```python
from build123d import *

# Parameters (mm, degrees)
SKETCH1_R           = 1.190625
SKETCH1_R_2         = 0.79375
BOSS_EXTRUDE1_DEPTH = 1.984375
SKETCH2_R           = 3.175
CUT_EXTRUDE1_DEPTH  = 0.7493
SKETCH3_R           = 4.365625
BOSS_EXTRUDE2_DEPTH = 2.3876
SKETCH4_R           = 2.778125
CUT_EXTRUDE2_DEPTH  = 2.9591
SKETCH5_R           = 3.7703125
SKETCH5_R_2         = 3.175
BOSS_EXTRUDE3_DEPTH = 0.4572


with BuildPart() as part:
    # Sketch1 → Boss-Extrude1 (new body)
    with BuildSketch(Plane(origin=(0, 0, 0), x_dir=(1, 0, 0), z_dir=(0, 1, 0))):
        with BuildLine():
            Line((-3.96335347, 4.938233395), (-2.375942501, 13.151798758))
            ThreePointArc((-2.375942501, 13.151798758), (-0.037956575, 15.081193279), (2.300029351, 13.151798758))
            Line((2.300029351, 13.151798758), (3.933761069, 4.9618349))
            ThreePointArc((3.933761069, 4.9618349), (4.283887399, 4.309571692), (4.938233395, 3.96335347))
            Line((4.938233395, 3.96335347), (13.151798758, 2.375942501))
            ThreePointArc((13.151798758, 2.375942501), (15.081193279, 0.037956575), (13.151798758, -2.300029351))
            Line((13.151798758, -2.300029351), (4.9618349, -3.933761069))
            ThreePointArc((4.9618349, -3.933761069), (4.309571692, -4.283887399), (3.96335347, -4.938233395))
            Line((3.96335347, -4.938233395), (2.375942501, -13.151798758))
            ThreePointArc((2.375942501, -13.151798758), (0.037956575, -15.081193279), (-2.300029351, -13.151798758))
            Line((-2.300029351, -13.151798758), (-3.933761069, -4.9618349))
            ThreePointArc((-3.933761069, -4.9618349), (-4.283887399, -4.309571692), (-4.938233395, -3.96335347))
            Line((-4.938233395, -3.96335347), (-13.151798758, -2.375942501))
            ThreePointArc((-13.151798758, -2.375942501), (-15.081193279, -0.037956575), (-13.151798758, 2.300029351))
            Line((-13.151798758, 2.300029351), (-4.9618349, 3.933761069))
            ThreePointArc((-4.9618349, 3.933761069), (-4.309571692, 4.283887399), (-3.96335347, 4.938233395))
        make_face()
        Circle(SKETCH1_R, mode=Mode.SUBTRACT)
        with Locations((-0.037956575, 12.699943279)):
            Circle(SKETCH1_R_2, mode=Mode.SUBTRACT)
        with Locations((-0.031124391, 10.413953489)):
            Circle(SKETCH1_R_2, mode=Mode.SUBTRACT)
        with Locations((-0.024292208, 8.127963699)):
            Circle(SKETCH1_R_2, mode=Mode.SUBTRACT)
        with Locations((12.699943279, 0.037956575)):
            Circle(SKETCH1_R_2, mode=Mode.SUBTRACT)
        with Locations((10.413953489, 0.031124391)):
            Circle(SKETCH1_R_2, mode=Mode.SUBTRACT)
        with Locations((8.127963699, 0.024292208)):
            Circle(SKETCH1_R_2, mode=Mode.SUBTRACT)
        with Locations((0.037956575, -12.699943279)):
            Circle(SKETCH1_R_2, mode=Mode.SUBTRACT)
        with Locations((0.031124391, -10.413953489)):
            Circle(SKETCH1_R_2, mode=Mode.SUBTRACT)
        with Locations((0.024292208, -8.127963699)):
            Circle(SKETCH1_R_2, mode=Mode.SUBTRACT)
        with Locations((-12.699943279, -0.037956575)):
            Circle(SKETCH1_R_2, mode=Mode.SUBTRACT)
        with Locations((-10.413953489, -0.031124391)):
            Circle(SKETCH1_R_2, mode=Mode.SUBTRACT)
        with Locations((-8.127963699, -0.024292208)):
            Circle(SKETCH1_R_2, mode=Mode.SUBTRACT)
    extrude(amount=BOSS_EXTRUDE1_DEPTH)

    # Sketch2 → Cut-Extrude1 (cut)
    with BuildSketch(Plane(origin=(0, 1.984375, 0), x_dir=(1, 0, 0), z_dir=(0, 1, 0))):
        Circle(SKETCH2_R)
    extrude(amount=-CUT_EXTRUDE1_DEPTH, mode=Mode.SUBTRACT)

    # Sketch3 → Boss-Extrude2 (add)
    with BuildSketch(Plane.XZ):
        Circle(SKETCH3_R)
    extrude(amount=BOSS_EXTRUDE2_DEPTH)

    # Sketch4 → Cut-Extrude2 (cut)
    with BuildSketch(Plane.XZ.offset(2.3876)):
        Circle(SKETCH4_R)
    extrude(amount=-CUT_EXTRUDE2_DEPTH, mode=Mode.SUBTRACT)

    # Sketch5 → Boss-Extrude3 (add)
    with BuildSketch(Plane(origin=(0, 1.984375, 0), x_dir=(1, 0, 0), z_dir=(0, 1, 0))):
        Circle(SKETCH5_R)
        Circle(SKETCH5_R_2, mode=Mode.SUBTRACT)
    extrude(amount=BOSS_EXTRUDE3_DEPTH)


solid = part.part
```
Model file for the job. Use its own axes, mm. A direction names the side the tool comes from. Give positions to 0.01 mm unless a question says otherwise; leave off trailing zeros. Write each loop counter-clockwise with the first axis right and the second up, starting at its lowest first coordinate (ties: lowest second). Pieces come first, ordered by that corner, then holes. Notation, with made-up numbers: (37, 17.5) - (46, 17.5) arc R22 cw to (46, 56.5) - close; hole circle Ø8 at (65.5, 29). An arc over 180 degrees is marked (long way). One line per question, with ' | ' between items. Start each with the question number.
(1) Slice it at D-D on x = 0. Give the number of separate pieces and of enclosed holes in the cut face, plus the area to 3 significant figures.
(2) Two-plate mould, pull along X, no slides. Class faces 3 (the face through (-3.767, 2.21, -0.166)), 4 (the face through (1.4, 1.235, 0)), 5 (the face through (-4.317, 0.978, -4.276)), 6 (the face through (8.99, 0.98, -3.18)): +X half, -X half, draft (parallel to the pull), parting line (faces both ways), or undercut.
(3) Pin check, flat tips, straight feed: P1, Ø1.5, axis at y = 0.5, z = 9.5, coming from the -X side; P2, Ø2, axis at x = 0.04, z = 12.7, coming from the -Y side; P3, Ø2, axis at x = -1, z = 5.5, coming from the +Y side. Stop position of each tip, or through.
(4) Slice it at A-A on z = -8.5. Write the cut outline in (x, y).
(5) Slice it at C-C on y = -1.8. Write the cut outline in (x, z), plus the area to 3 significant figures.
(6) 3-axis set-ups, long thin cutter, end or side, ignore diameter. For faces 1 (the face through (1, 0.571, -1)), 2 (the face through (-9.657, 0.978, -0.207)): which of +Z, -Z, +X, -X, +Y, -Y reach the whole face in a straight line?
(7) Wall check: line 1 along Z through (x, y) = (0, 2.1) (3 decimals); line 2 along Y through (x, z) = (13.5, -1.5); line 3 along X through (y, z) = (-1.9, 2). Give the ranges that are in metal, low to high. Write a range as from..to.
(8) Slice it at B-B on x = -10. Write the cut outline in (y, z).
Results below:
1) separate pieces: 8 | enclosed holes: 0 | area: 39.6 mm^2
2) face 3: parting line | face 4: undercut | face 5: -X half | face 6: +X half
3) P1: x = -3.18 | P2: y = 0 | P3: y = 1.98
4) outline: (-3.27, 0) - (-0.73, 0) - (-0.73, 1.98) - (-3.27, 1.98) - close; (0.68, 0) - (3.23, 0) - (3.23, 1.98) - (0.68, 1.98) - close
5) outline: circle Ø8.73 at (0, 0); hole circle Ø5.56 at (0, 0) | area: 35.6 mm^2
6) face 1: -Y | face 2: +Y, -Y
7) line 1: -3.77..-3.175, 3.175..3.77 | line 2: 0..1.98 | line 3: -3.88..-1.93, 1.93..3.88
8) outline: (0, -2.93) - (1.98, -2.93) - (1.98, -0.65) - (0, -0.65) - close; (0, 0.71) - (1.98, 0.71) - (1.98, 2.99) - (0, 2.99) - close
